The figure shows three views and two pictorial views of one solid part (mm, origin at its lowest corner). Answer the questions. Round coordinates to 2 decimals unless told otherwise and drop trailing zeros. Order: outer loops, then holes, each group sorted by start corner. A loop starts at its lowest first (then second) coordinate and runs counter-clockwise, first axis right, second up. Notation, with made-up numbers: (-11.5, -25) -> (35.5, -25) arc R20 cw to (35.5, 11) -> close; hole circle Ø11 at (-32, 55.5). An arc over 180 degrees is marked (long way). Answer as a JSON object with one key per item and string values. Group by question number.
Item 1: Section A-A, the plane x = 1132.5 is taken. Write down the section's boundary in (y, z).
Item 2: Section C-C, the plane z = 5.25 is taken. Write down the section's boundary in (x, y).
Item 3: Section B-B, the plane y = 263.5 is taken. Write down the section's boundary in (x, z).
Item 4: Given P1, Ø12, axis at x = 409.5, y = 376, coming from the -Z side, flat-ended and moving along its own axis, determine where the tip first touches the part or whether it passes through.
Item 5: Consider probe 1 along X at (y, z) = (333.5, 17.75); probe 2 along Y at (x, z) = (943.5, 17). Determine where each line is inside the solid, lowest interval first. Write a range as from..to.
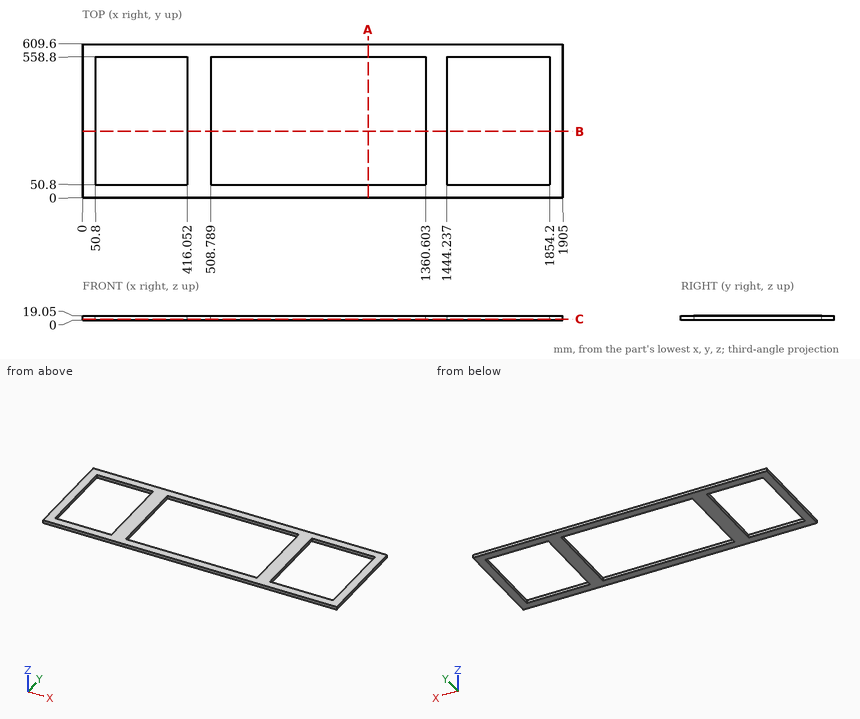
Values found:
{
 "1": {"outline": "(0, 0) -> (50.8, 0) -> (50.8, 19.05) -> (0, 19.05) -> close; (558.8, 0) -> (609.6, 0) -> (609.6, 19.05) -> (558.8, 19.05) -> close"},
 "2": {"outline": "(0, 0) -> (1905, 0) -> (1905, 609.6) -> (0, 609.6) -> close; hole (50.8, 50.8) -> (416.05, 50.8) -> (416.05, 558.8) -> (50.8, 558.8) -> close; hole (508.79, 50.8) -> (1360.6, 50.8) -> (1360.6, 558.8) -> (508.79, 558.8) -> close; hole (1444.24, 50.8) -> (1854.2, 50.8) -> (1854.2, 558.8) -> (1444.24, 558.8) -> close"},
 "3": {"outline": "(0, 0) -> (50.8, 0) -> (50.8, 19.05) -> (0, 19.05) -> close; (416.05, 0) -> (508.79, 0) -> (508.79, 19.05) -> (416.05, 19.05) -> close; (1360.6, 0) -> (1444.24, 0) -> (1444.24, 19.05) -> (1360.6, 19.05) -> close; (1854.2, 0) -> (1905, 0) -> (1905, 19.05) -> (1854.2, 19.05) -> close"},
 "4": {"P1": "through"},
 "5": {"probe 1": "0..50.8, 416.05..508.79, 1360.6..1444.24, 1854.2..1905", "probe 2": "0..50.8, 558.8..609.6"}
}
